CAD build for the part. Positions are in the model's coordinates, mm. A direction names the side the tool comes from. Round coordinates to 2 decimals unless told otherwise and drop trailing zeros. Order: outer loops, then holes, each group sorted by start corner. A loop starts at its lowest first (then second) coordinate and runs counter-clockwise, first axis right, second up. Notation, with made-up numbers: M -22,-39 L 11,-39 A7 ccw 11,-29 Z; hole C 74,-2 d1. An arc over 180 degrees is marked long. Answer as a JSON object with one key per item and string values.
```python
from build123d import *

# Parameters (mm, degrees)
SKETCH1_W           = 100
SKETCH1_H           = 150
BOSS_EXTRUDE1_DEPTH = 20
SKETCH2_R           = 5.25
CUT_EXTRUDE1_DEPTH  = 26
SKETCH3_W           = 4.7
SKETCH3_H           = 150
CUT_EXTRUDE2_DEPTH  = 20


with BuildPart() as part:
    # Sketch1 → Boss-Extrude1 (new body)
    with BuildSketch(Plane.XY):
        with Locations((-49.435028249, 17.09039548)):
            Rectangle(SKETCH1_W, SKETCH1_H)
    extrude(amount=BOSS_EXTRUDE1_DEPTH)

    # Sketch2 → Cut-Extrude1 (cut)
    with BuildSketch(Plane(origin=(0, 92.09039548, 0), x_dir=(1, 0, 0), z_dir=(0, 1, 0))):
        with Locations(Location((-58.935028249, -10, 0), (0, 0, 270))):
            Circle(SKETCH2_R)
        with Locations(Location((-39.935028249, -10, 0), (0, 0, 270))):
            Circle(SKETCH2_R)
    extrude(amount=-CUT_EXTRUDE1_DEPTH, mode=Mode.SUBTRACT)

    # Sketch3 → Cut-Extrude2 (cut)
    with BuildSketch(Plane.XY.offset(20)):
        with Locations((-97.085028249, 17.09039548)):
            Rectangle(SKETCH3_W, SKETCH3_H)
        with Locations((-1.785028249, 17.09039548)):
            Rectangle(SKETCH3_W, SKETCH3_H)
    extrude(amount=-CUT_EXTRUDE2_DEPTH, mode=Mode.SUBTRACT)


solid = part.part
```
Item 1: 3-axis set-ups, long thin cutter, end or side, ignore diameter. For faces 5 (the flat face through (-59, 66.09, 10)), 6 (the flat face through (-50, 18, 20)): which of +Z, -Z, +X, -X, +Y, -Y reach the whole face in a straight line?
Worked answers:
{"face 5": "+Y", "face 6": "+Z, +X, -X, +Y, -Y"}
Item 2: Drop a flat-ended pin along its axis: pin 1 Ø8.5 at (x, z) = (-58.94, 10) entering from +Y. Give the stop position or say it passes through.
Worked answers:
{"pin 1": "stops at y = 66.09"}
Item 3: Wall check: line 1 along X through (y, z) = (81.5, 10); line 2 along X through (y, z) = (79.5, 11.25); line 3 along Y through (x, z) = (-37, 10). Give the ranges that are in metal, low to high. Write a range as [from, to].
Worked answers:
{"line 1": "x = [-94.74, -64.19], [-53.69, -45.19], [-34.69, -4.14]", "line 2": "x = [-94.74, -64.03], [-53.84, -45.03], [-34.84, -4.14]", "line 3": "y = [-57.91, 66.09]"}
Item 4: Two-plate mould, pull along X, no slides. Class faces 1 (the flat face through (-4.135, 16, 10)), 2 (the flat face through (-94.735, 16, 10)), 3 (the flat face through (-50, 92.09, 10)), 4 (the cylindrical face through (-54.508, 79.272, 12.822)): released by +X, released by -X, zero draft, split by the parting line, or undercut.
Worked answers:
{"face 1": "released by +X", "face 2": "released by -X", "face 3": "zero draft", "face 4": "undercut"}
Item 5: Saw through at A-A on z = 10. List the corners of the cut face in (x, y).
Worked answers:
{"outline": "M -94.74,-57.91 L -4.14,-57.91 L -4.14,92.09 L -34.69,92.09 L -34.69,66.09 L -45.19,66.09 L -45.19,92.09 L -53.69,92.09 L -53.69,66.09 L -64.19,66.09 L -64.19,92.09 L -94.74,92.09 Z"}
Item 6: Saw through at B-B on x = -56. List the corners of the cut face in (y, z).
Worked answers:
{"outline": "M -57.91,0 L 92.09,0 L 92.09,5.65 L 66.09,5.65 L 66.09,14.35 L 92.09,14.35 L 92.09,20 L -57.91,20 Z"}
